Source: three-view drawing plus pictorial views. Frame: mm from the lowest corner of the part. Round coordinates to 2 decimals unless told otherwise and drop trailing zeros. Write each loop counter-clockwise with the first axis right and the second up, starting at its lowest first coordinate (ties: lowest second). Pieces come first, ordered by that corner, then holes. Notation, with made-up numbers: M 49.5,51 L 90.5,51 A25 ccw 90.5,71 Z; hole C -38.75,-12.75 d3. An arc over 180 degrees is marked long. Answer as CSV lines item,"result". Start each with the question number.
Q1. Ray query, probe 1 along X at (y, z) = (4.75, 43.5); probe 2 along X at (y, z) = (4.75, 47.5). Return the intervals inside material, ascending.
Q2. Section query A-A on z = 13. Output: boundary loops of the cut face in (x, y), and give its area (3 significant figures).
Q3. Section query B-B on y = 4.75. Output: boundary loops of the cut face in (x, z).
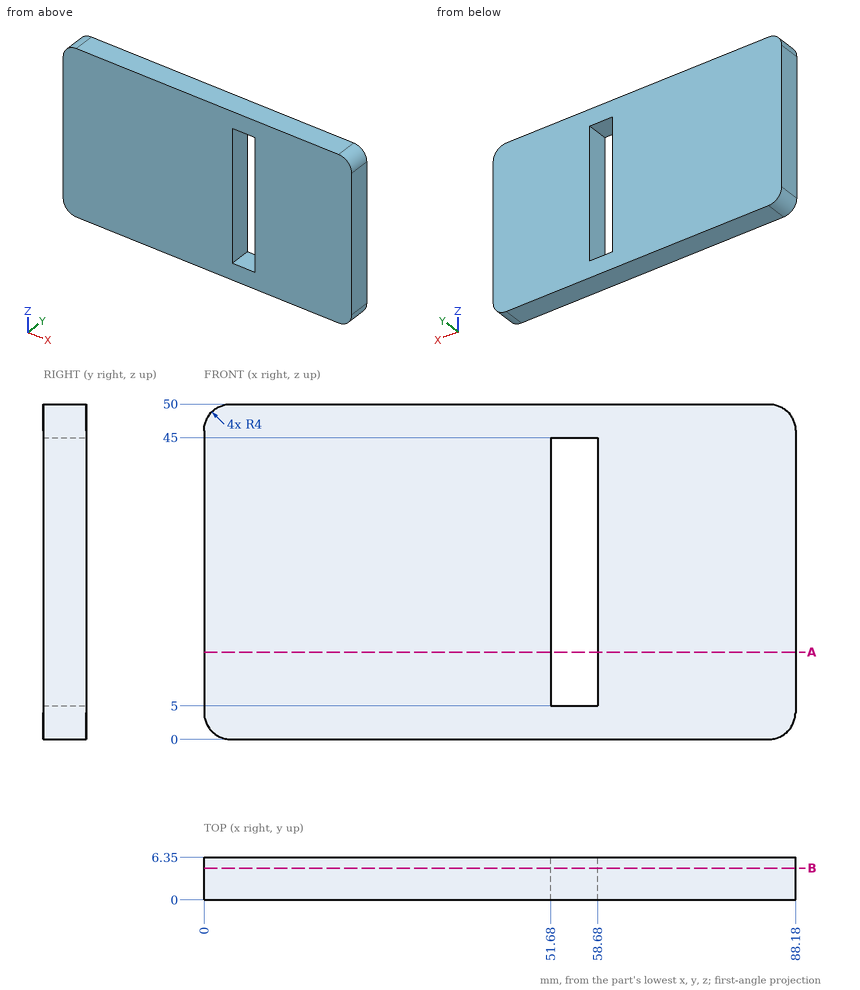
Entries:
1,probe 1,"x = 0 to 51.68, 58.68 to 88.18"
1,probe 2,"x = 0.29 to 87.89"
2,outline,"M 0,0 L 51.68,0 L 51.68,6.35 L 0,6.35 Z; M 58.68,0 L 88.18,0 L 88.18,6.35 L 58.68,6.35 Z"
2,area,"515 mm^2"
3,outline,"M 0,4 A4 ccw 4,0 L 84.18,0 A4 ccw 88.18,4 L 88.18,46 A4 ccw 84.18,50 L 4,50 A4 ccw 0,46 Z; hole M 51.68,5 L 58.68,5 L 58.68,45 L 51.68,45 Z"
